Part model, mm, in its own coordinate system. A direction names the side the tool comes from. Coordinates: 2 decimals unless noted, no trailing zeros. Write each loop counter-clockwise with the first axis right and the second up, starting at its lowest first coordinate (ties: lowest second). Pieces come first, ordered by that corner, then holes. Notation, with made-up numbers: M 51.5,-33 L 64.5,-33 A14 ccw 64.5,-12 Z; hole C -15,-24 d7. An arc over 180 degrees is marked long. Use a Markdown table: item, result. Add a question column.
Q1. Slice it at D-D on y = 88.5. Write the cut outline in (x, z).
Q2. Slice it at A-A on x = -85. Write the cut outline in (y, z).
Q3. Mould opens along X. For faces 3 (the flat face through (-94, 82, 5)), 4 (the flat face through (-82.477, 81.43, 3.014)), 5 (the cylindrical face through (-79.62, 88.43, 2.46)) say: released by +X, released by -X, zero draft, split by the parting line, or undercut.
Q4. Slice it at C-C on x = -93.5. Write the cut outline in (y, z), then the cut area to 3 significant figures.
Q5. Tool access for faces 1 (the flat face through (-85, 78, 0)), 2 (the flat face through (-87, 81, 2)): list every direction of +Z, -Z, +X, -X, +Y, -Y with a clear straight run to the whole face (end or side of a thin tool).
Q6. Slice it at B-B on z = 4.5. Write the cut outline in (x, y).
Q7. Wall check: L1, parallel to Y at x = -85, z = 4.35; L2, parallel to Y at x = -85, z = 0.95; L3, parallel to Z at x = -88.5, y = 77.75. Give the ranges that are in metal, low to high. Write a range as from..to.
Q8. Pin check, flat tips, straight feed: pin 1 Ø3 at (x, y) = (-85.5, 78.5) entering from +Z; pin 2 Ø1 at (x, z) = (-86, 4.5) entering from -Y; pin 3 Ø1.5 at (y, z) = (74, 3) entering from +X. Stop position of each tip, or through.
from build123d import *

# Parameters (mm, degrees)
SKETCH1_R           = 10
SKETCH1_R_2         = 1.5
BOSS_EXTRUDE1_DEPTH = 2
SKETCH2_R           = 10
SKETCH2_R_2         = 1.5
BOSS_EXTRUDE2_DEPTH = 3
SKETCH3_R           = 1.6
CUT_EXTRUDE1_DEPTH  = 131.958008585
CUT_EXTRUDE2_DEPTH  = 3
SKETCH5_R           = 9
CUT_EXTRUDE3_DEPTH  = 1


with BuildPart() as part:
    # Sketch1 → Boss-Extrude1 (new body)
    with BuildSketch(Plane.XY):
        with Locations((-85.000000067, 80)):
            Circle(SKETCH1_R)
        with Locations((-85.000000067, 80)):
            Circle(SKETCH1_R_2, mode=Mode.SUBTRACT)
    extrude(amount=BOSS_EXTRUDE1_DEPTH)

    # Sketch2 → Boss-Extrude2 (add)
    # profile 1 of 2: a face of its own
    with BuildSketch(Plane.XY.offset(2)):
        with Locations((-85.000000067, 80)):
            Circle(SKETCH2_R)
        with Locations((-85.000000067, 80)):
            Circle(SKETCH2_R_2, mode=Mode.SUBTRACT)
    # profile 2 of 2: a face of its own
    with BuildSketch(Plane.XY.offset(2)):
        with Locations((-85.000000067, 80)):
            Circle(SKETCH2_R_2)
    extrude(amount=BOSS_EXTRUDE2_DEPTH)

    # Sketch3 → Cut-Extrude1 (cut, through all)
    with BuildSketch(Plane(origin=(0, 0, 0), x_dir=(-1, 0, 0), z_dir=(0, 0, -1))):
        with Locations((85.000000067, 80)):
            Circle(SKETCH3_R)
    extrude(amount=-CUT_EXTRUDE1_DEPTH, mode=Mode.SUBTRACT)

    # Sketch4 → Cut-Extrude2 (cut)
    with BuildSketch(Plane.XY.offset(5)):
        Polygon((-88.348631628, 80), (-86.674315847, 77.1), (-83.325684286, 77.1), (-81.651368505, 80), (-83.325684286, 82.9), (-86.674315847, 82.9), align=None)
    extrude(amount=-CUT_EXTRUDE2_DEPTH, mode=Mode.SUBTRACT)

    # Sketch5 → Cut-Extrude3 (cut)
    with BuildSketch(Plane.XY.offset(5)):
        with Locations((-85.000000067, 80)):
            Circle(SKETCH5_R)
    extrude(amount=-CUT_EXTRUDE3_DEPTH, mode=Mode.SUBTRACT)


solid = part.part
Recorded:
| question | item | result |
|---|---|---|
| 1 | outline | M -90.27,0 L -79.73,0 L -79.73,5 L -82.04,5 L -82.04,4 L -87.96,4 L -87.96,5 L -90.27,5 Z |
| 2 | outline | M 70,0 L 78.4,0 L 78.4,2 L 77.1,2 L 77.1,4 L 71,4 L 71,5 L 70,5 Z; M 81.6,0 L 90,0 L 90,5 L 89,5 L 89,4 L 82.9,4 L 82.9,2 L 81.6,2 Z |
| 3 | face 3 | zero draft |
| 3 | face 4 | undercut |
| 3 | face 5 | split by the parting line |
| 4 | outline | M 74.73,0 L 85.27,0 L 85.27,5 L 82.96,5 L 82.96,4 L 77.04,4 L 77.04,5 L 74.73,5 Z |
| 4 | area | 46.8 mm² |
| 5 | face 1 | -Z, +X, -X, +Y, -Y |
| 5 | face 2 | +Z |
| 6 | outline | C -85,80 d20; hole C -85,80 d18 |
| 7 | L1 | 70..71, 89..90 |
| 7 | L2 | 70..78.4, 81.6..90 |
| 7 | L3 | 0..4 |
| 8 | pin 1 | z = 4 |
| 8 | pin 2 | y = 70.01 |
| 8 | pin 3 | x = -76.49 |
